Verification items for the finished model (mm, model axes). Coordinates: 2 decimals unless noted, no trailing zeros. Order: outer loops, then holes, each group sorted by start corner. A loop starts at its lowest first (then second) coordinate and runs counter-clockwise, first axis right, second up. Notation, with made-up numbers: (52.25, 62.5) -> (92.25, 62.5) arc R19 cw to (92.25, 68.5) -> close; hole circle Ø10 at (52, -32.75). An arc over 180 degrees is marked (long way). Use CSV: the item, a comma, the result in double quotes. Start each with the question number.
1) Sectioned sample at B-B on z = 0.75. Give the number of separate pieces and of enclosed holes in the cut face, then the cut area to 3 significant figures.
2) Go/stop test with flat-tipped pins: pin 1 (0.9 mm diameter, centred on y = -174.5, z = 1, fed in from +X); pin 2 (0.9 mm diameter, centred on y = 99, z = 1.5, fed in from -X). Record where each tip stops, or that it passes through.
3) Scan lines: line 1 along Y through (x, z) = (148.5, 2); line 2 along Y through (x, z) = (-176, 1.5); line 3 along X through (y, z) = (-96.5, 0.75). Record each from-to range of solid material in increasing order.
4) Sectioned sample at A-A on x = -166. Record the boundary of the cut face in (y, z).
from build123d import *

# Parameters (mm, degrees)
CROQUIS1_W              = 600
CROQUIS1_H              = 500
CROQUIS1_R              = 5
SALIENTE_EXTRUIR1_DEPTH = 3
CROQUIS5_W              = 49.8
CROQUIS5_H              = 3
CROQUIS5_W_2            = 3
CROQUIS5_H_2            = 44.8
CORTAR_EXTRUIR2_DEPTH   = 4


with BuildPart() as part:
    # Croquis1 → Saliente-Extruir1 (new body)
    with BuildSketch(Plane.XY):
        Rectangle(CROQUIS1_W, CROQUIS1_H)
        with Locations((-250, -200)):
            Circle(CROQUIS1_R, mode=Mode.SUBTRACT)
        with Locations((-250, -6.5)):
            Circle(CROQUIS1_R, mode=Mode.SUBTRACT)
        with Locations((250, -200)):
            Circle(CROQUIS1_R, mode=Mode.SUBTRACT)
        with Locations((250, -6.5)):
            Circle(CROQUIS1_R, mode=Mode.SUBTRACT)
        with BuildLine():
            Line((-250, 201), (-50, 201))
            ThreePointArc((-50, 201), (-46, 197), (-50, 193))
            Line((-50, 193), (-250, 193))
            ThreePointArc((-250, 193), (-254, 197), (-250, 201))
        make_face(mode=Mode.SUBTRACT)
        with BuildLine():
            Line((-250, 117), (-50, 117))
            ThreePointArc((-50, 117), (-46, 121), (-50, 125))
            Line((-50, 125), (-250, 125))
            ThreePointArc((-250, 125), (-254, 121), (-250, 117))
        make_face(mode=Mode.SUBTRACT)
        with BuildLine():
            Line((-250, -111), (-50, -111))
            ThreePointArc((-50, -111), (-46, -107), (-50, -103))
            Line((-50, -103), (-250, -103))
            ThreePointArc((-250, -103), (-254, -107), (-250, -111))
        make_face(mode=Mode.SUBTRACT)
        with BuildLine():
            Line((-250, -187), (-50, -187))
            ThreePointArc((-50, -187), (-46, -183), (-50, -179))
            Line((-50, -179), (-250, -179))
            ThreePointArc((-250, -179), (-254, -183), (-250, -187))
        make_face(mode=Mode.SUBTRACT)
        with BuildLine():
            Line((250, -103), (50, -103))
            ThreePointArc((50, -103), (46, -107), (50, -111))
            Line((50, -111), (250, -111))
            ThreePointArc((250, -111), (254, -107), (250, -103))
        make_face(mode=Mode.SUBTRACT)
        with BuildLine():
            Line((250, -179), (50, -179))
            ThreePointArc((50, -179), (46, -183), (50, -187))
            Line((50, -187), (250, -187))
            ThreePointArc((250, -187), (254, -183), (250, -179))
        make_face(mode=Mode.SUBTRACT)
        with BuildLine():
            Line((250, 201), (50, 201))
            ThreePointArc((50, 201), (46, 197), (50, 193))
            Line((50, 193), (250, 193))
            ThreePointArc((250, 193), (254, 197), (250, 201))
        make_face(mode=Mode.SUBTRACT)
        with BuildLine():
            Line((250, 125), (50, 125))
            ThreePointArc((50, 125), (46, 121), (50, 117))
            Line((50, 117), (250, 117))
            ThreePointArc((250, 117), (254, 121), (250, 125))
        make_face(mode=Mode.SUBTRACT)
    extrude(amount=SALIENTE_EXTRUIR1_DEPTH)

    # Croquis5 → Cortar-Extruir2 (cut, through all)
    with BuildSketch(Plane(origin=(0, 0, 0), x_dir=(-1, 0, 0), z_dir=(0, 0, -1))):
        with Locations((150, 248.5)):
            Rectangle(CROQUIS5_W, CROQUIS5_H)
        with Locations((50, 248.5)):
            Rectangle(CROQUIS5_W, CROQUIS5_H)
        with Locations((250, 248.5)):
            Rectangle(CROQUIS5_W, CROQUIS5_H)
        with Locations((-50, 248.5)):
            Rectangle(CROQUIS5_W, CROQUIS5_H)
        with Locations((-150, 248.5)):
            Rectangle(CROQUIS5_W, CROQUIS5_H)
        with Locations((298.5, 180)):
            Rectangle(CROQUIS5_W_2, CROQUIS5_H_2)
        with Locations((-250, 248.5)):
            Rectangle(CROQUIS5_W, CROQUIS5_H)
        with Locations((298.5, 90)):
            Rectangle(CROQUIS5_W_2, CROQUIS5_H_2)
        with Locations((298.5, 0)):
            Rectangle(CROQUIS5_W_2, CROQUIS5_H_2)
        with Locations((298.5, -90)):
            Rectangle(CROQUIS5_W_2, CROQUIS5_H_2)
        with Locations((298.5, -180)):
            Rectangle(CROQUIS5_W_2, CROQUIS5_H_2)
        with Locations((-250, -248.5)):
            Rectangle(CROQUIS5_W, CROQUIS5_H)
        with Locations((-150, -248.5)):
            Rectangle(CROQUIS5_W, CROQUIS5_H)
        with Locations((-50, -248.5)):
            Rectangle(CROQUIS5_W, CROQUIS5_H)
        with Locations((50, -248.5)):
            Rectangle(CROQUIS5_W, CROQUIS5_H)
        with Locations((250, -248.5)):
            Rectangle(CROQUIS5_W, CROQUIS5_H)
        with Locations((150, -248.5)):
            Rectangle(CROQUIS5_W, CROQUIS5_H)
        with Locations((-298.5, -180)):
            Rectangle(CROQUIS5_W_2, CROQUIS5_H_2)
        with Locations((-298.5, -90)):
            Rectangle(CROQUIS5_W_2, CROQUIS5_H_2)
        with Locations((-298.5, 0)):
            Rectangle(CROQUIS5_W_2, CROQUIS5_H_2)
        with Locations((-298.5, 90)):
            Rectangle(CROQUIS5_W_2, CROQUIS5_H_2)
        with Locations((-298.5, 180)):
            Rectangle(CROQUIS5_W_2, CROQUIS5_H_2)
    extrude(amount=-CORTAR_EXTRUIR2_DEPTH, mode=Mode.SUBTRACT)


solid = part.part
Answers follow:
1,separate pieces,"1"
1,enclosed holes,"12"
1,area,"283,000 mm²"
2,pin 1,"stops at x = 297"
2,pin 2,"stops at x = -297"
3,line 1,"y = -247 to -187, -179 to -111, -103 to 117, 125 to 193, 201 to 247"
3,line 2,"y = -250 to -187, -179 to -111, -103 to 117, 125 to 193, 201 to 250"
3,line 3,"x = -297 to 297"
4,outline,"(-247, 0) -> (-187, 0) -> (-187, 3) -> (-247, 3) -> close; (-179, 0) -> (-111, 0) -> (-111, 3) -> (-179, 3) -> close; (-103, 0) -> (117, 0) -> (117, 3) -> (-103, 3) -> close; (125, 0) -> (193, 0) -> (193, 3) -> (125, 3) -> close; (201, 0) -> (247, 0) -> (247, 3) -> (201, 3) -> close"
